Source: three-view drawing plus pictorial views. Frame: mm from the lowest corner of the part. A direction names the side the tool comes from. Give positions to 0.01 mm unless a question says otherwise; leave off trailing zeros. Loops run counter-clockwise (first coordinate to the right, second up) from the corner with the lowest first, then second, coordinate; pieces in that order, holes last. Notation, with made-up numbers: (3.25, -11) - (52.25, -11) arc R32 ccw to (52.25, 23) - close; hole circle Ø2 at (89.5, 38.5). An arc over 180 degrees is marked (long way). Answer as a JSON object with one key per item and string values.
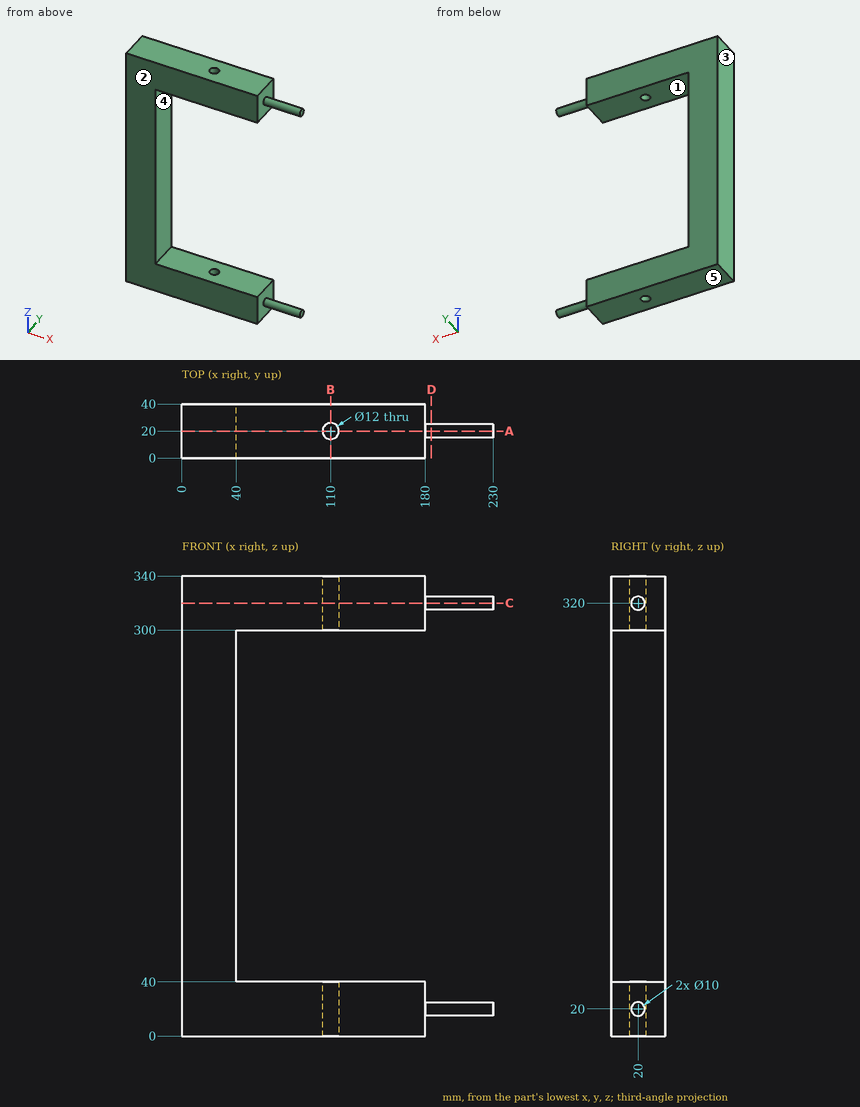
Item 1: Material intervals for line 1 (Z direction, x = 88.5, y = 38); line 2 (Y direction, x = 110, z = 26); line 3 (X direction, y = 27, z = 286.5), sorted ascending. Write a range as [from, to].
Geometry check:
{"line 1": "z = [0, 40], [300, 340]", "line 2": "y = [0, 14], [26, 40]", "line 3": "x = [0, 40]"}
Item 2: Cut plane C-C (z = 320). Return loops of the section in (x, y), then the cut area to 3 significant figures.
Geometry check:
{"outline": "(0, 0) - (180, 0) - (180, 15) - (230, 15) - (230, 25) - (180, 25) - (180, 40) - (0, 40) - close; hole circle Ø12 at (110, 20)", "area": "7,590 mm2"}
Item 3: Access query for the marked faces 1 and 2. Directions: +Z, -Z, +X, -X, +Y, -Y. A direction counts if a zero-diameter tool reaches every point of the face in a straight line with its end or side. Return the directions, or none.
Geometry check:
{"face 1": "+X, +Y, -Y", "face 2": "+Z, -Z, +X, -X, -Y"}
Item 4: Cut plane B-B (x = 110). Return loops of the section in (y, z), then the cut area to 3 significant figures.
Geometry check:
{"outline": "(0, 0) - (14, 0) - (14, 40) - (0, 40) - close; (0, 300) - (14, 300) - (14, 340) - (0, 340) - close; (26, 0) - (40, 0) - (40, 40) - (26, 40) - close; (26, 300) - (40, 300) - (40, 340) - (26, 340) - close", "area": "2,240 mm2"}
Item 5: Mould query, pull axis Z, two halves, no side actions, for the marked faces 3, 4 and 5. Classes: released by +Z, released by -Z, zero draft, split by the parting line, or undercut.
Geometry check:
{"face 3": "zero draft", "face 4": "undercut", "face 5": "released by -Z"}
Item 6: Cut plane A-A (y = 20). Return loops of the section in (x, z).
Geometry check:
{"outline": "(0, 0) - (104, 0) - (104, 40) - (40, 40) - (40, 300) - (104, 300) - (104, 340) - (0, 340) - close; (116, 0) - (180, 0) - (180, 15) - (230, 15) - (230, 25) - (180, 25) - (180, 40) - (116, 40) - close; (116, 300) - (180, 300) - (180, 315) - (230, 315) - (230, 325) - (180, 325) - (180, 340) - (116, 340) - close"}
Item 7: Contact query for flat-ended pins moving along their axis: P1, Ø1.5, axis at y = 14.5, z = 246.5, coming from the +X side; P2, Ø12, axis at y = 26.5, z = 10.5, coming from the +X side. Output: stop coordinate, or through.
Geometry check:
{"P1": "stops at x = 40", "P2": "stops at x = 180"}
Item 8: Cut plane D-D (x = 184.5). Return loops of the section in (y, z), then the cut area to 3 significant figures.
Geometry check:
{"outline": "circle Ø10 at (20, 20); circle Ø10 at (20, 320)", "area": "157 mm2"}
